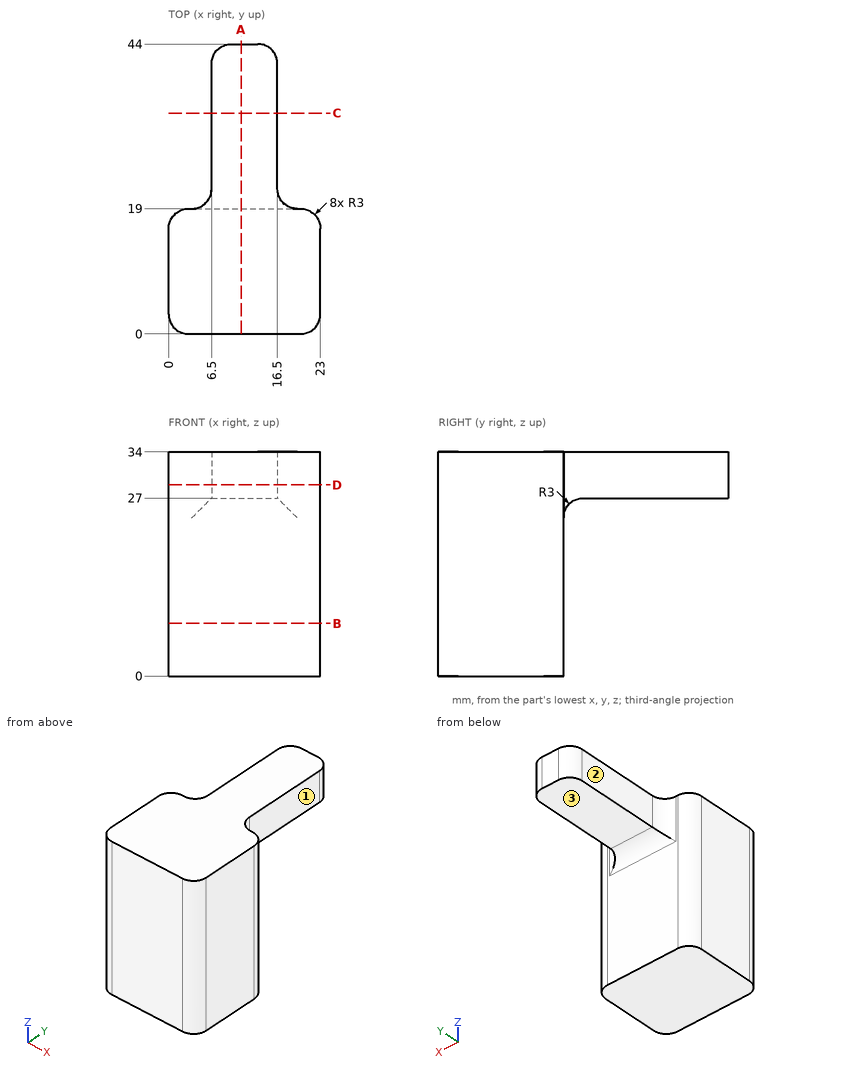
Job drawing, mm, ordinate dimensions from the low corner. One solid piece. A direction names the side the tool comes from. Give positions to 0.01 mm unless a question says otherwise; leave off trailing zeros. Write each loop counter-clockwise with the first axis right and the second up, starting at its lowest first coordinate (ties: lowest second). Pieces come first, ordered by that corner, then holes. Notation, with made-up numbers: (57.25, 29.25) - (79.25, 29.25) arc R7 ccw to (79.25, 34.25) - close; hole circle Ø11 at (10, -35). An arc over 180 degrees is marked (long way). Use one line per item in the form item = value. Start each with the question number.
1. Probe line 1 (Z direction, x = 11, y = 29); line 2 (Y direction, x = 9.5, z = 12); line 3 (X direction, y = 41, z = 27.5). List the from-to ranges inside material, lowest first. Write a range as [from, to].
2. Band-saw the part on C-C on y = 33.5. Write the cut outline in (x, z), plus the area to 3 significant figures.
3. Band-saw the part on B-B on z = 8. Write the cut outline in (x, y).
4. 3-axis set-ups, long thin cutter, end or side, ignore diameter. For the marked faces 1, 2 and 3: which of +Z, -Z, +X, -X, +Y, -Y reach the whole face in a straight line?
5. Band-saw the part on A-A on x = 11. Write the cut outline in (y, z), plus the area to 3 significant figures.
6. Band-saw the part on D-D on z = 29. Write the cut outline in (x, y), plus the area to 3 significant figures.
7. Drop flat-ended pins along their axis: pin 1 Ø1 at (x, z) = (11.5, 17) entering from +Y; pin 2 Ø7.5 at (y, z) = (32.5, 31) entering from +X; pin 3 Ø8.5 at (x, z) = (8, 22.5) entering from +Y. Give the stop position or say it passes through.
Conclusion:
q1.line_1 = [27, 34]
q1.line_2 = [0, 19]
q1.line_3 = [6.5, 16.5]
q2.outline = (6.5, 27) - (16.5, 27) - (16.5, 34) - (6.5, 34) - close
q2.area = 70.0 mm²
q3.outline = (0, 3) arc R3 ccw to (3, 0) - (20, 0) arc R3 ccw to (23, 3) - (23, 16) arc R3 ccw to (20, 19) - (3, 19) arc R3 ccw to (0, 16) - close
q4.face_1 = +Z, -Z, +X, +Y
q4.face_2 = +Z, -Z, -X, +Y
q4.face_3 = -Z, +X, -X, +Y
q5.outline = (0, 0) - (19, 0) - (19, 24) arc R3 cw to (22, 27) - (44, 27) - (44, 34) - (0, 34) - close
q5.area = 823 mm²
q6.outline = (0, 3) arc R3 ccw to (3, 0) - (20, 0) arc R3 ccw to (23, 3) - (23, 16) arc R3 ccw to (20, 19) - (19.5, 19) arc R3 cw to (16.5, 22) - (16.5, 41) arc R3 ccw to (13.5, 44) - (9.5, 44) arc R3 ccw to (6.5, 41) - (6.5, 22) arc R3 cw to (3.5, 19) - (3, 19) arc R3 ccw to (0, 16) - close
q6.area = 679 mm²
q7.pin_1 = 19
q7.pin_2 = 16.5
q7.pin_3 = 20.8
